from build123d import *

# Parameters (mm, degrees)
F0_W      = 1841.5
F0_H      = 622.3
F1_DEPTH  = 711.2
F2_W      = 1739.9
F2_H      = 609.6
F3_DEPTH  = 762
F4_W      = 520.7
F4_H      = 609.6
F5_DEPTH  = 2540
F6_W      = 1739.9
F6_H      = 520.7
F7_DEPTH  = 2540
F8_W      = 50.8
F8_H      = 50.8
F9_DEPTH  = 520.7
F10_W     = 50.8
F10_H     = 50.8
F11_DEPTH = 609.6
F12_W     = 50.8
F12_H     = 50.8
F13_DEPTH = 609.6


with BuildPart() as f1:
    # F0 (on Top) → F1 (new body)
    with BuildSketch(Plane.XY):
        with Locations((814.200432, 140.348346)):
            Rectangle(F0_W, F0_H)
    extrude(amount=F1_DEPTH)

    # F2 (on face) → F3 (cut)
    with BuildSketch(Plane.XZ.offset(170.801654)):
        with Locations((814.200432, 355.6)):
            Rectangle(F2_W, F2_H)
    extrude(amount=-F3_DEPTH, mode=Mode.SUBTRACT)

    # F4 (on face) → F5 (cut)
    with BuildSketch(Plane(origin=(-106.549568, 0, 0), x_dir=(0, -1, 0), z_dir=(-1, 0, 0))):
        with Locations((-140.348346, 355.6)):
            Rectangle(F4_W, F4_H)
    extrude(amount=-F5_DEPTH, mode=Mode.SUBTRACT)

    # F6 (on face) → F7 (cut)
    with BuildSketch(Plane.XY.offset(711.2)):
        with Locations((814.200432, 140.348346)):
            Rectangle(F6_W, F6_H)
    extrude(amount=-F7_DEPTH, mode=Mode.SUBTRACT)

    # F8 (on face) → F9 (join)
    with BuildSketch(Plane.XZ.offset(-400.698346)):
        with Locations((515.750432, 685.8)):
            Rectangle(F8_W, F8_H)
        with Locations((1112.650432, 685.8)):
            Rectangle(F8_W, F8_H)
    extrude(amount=F9_DEPTH)

    # F10 (on face) → F11 (join)
    with BuildSketch(Plane(origin=(0, 0, 660.4), x_dir=(1, 0, 0), z_dir=(0, 0, -1))):
        with Locations((1112.650432, -426.098346)):
            Rectangle(F10_W, F10_H)
        with Locations((515.750432, -426.098346)):
            Rectangle(F10_W, F10_H)
    extrude(amount=F11_DEPTH)

    # F12 (on face) → F13 (join)
    with BuildSketch(Plane(origin=(0, 0, 660.4), x_dir=(1, 0, 0), z_dir=(0, 0, -1))):
        with Locations((515.750432, 145.401654)):
            Rectangle(F12_W, F12_H)
        with Locations((1112.650432, 145.401654)):
            Rectangle(F12_W, F12_H)
    extrude(amount=F13_DEPTH)


solid = f1.part
Can you work these out from the model? Positions are in its coordinate system, mm. A direction names the side the tool comes from. Round coordinates to 2 decimals unless told otherwise and drop trailing zeros. Order: outer loops, then holes, each group sorted by start corner. A loop starts at its lowest first (then second) coordinate and runs counter-clockwise, first axis right, second up. Notation, with made-up numbers: M 85,15 L 103,15 A22 ccw 103,43 Z; hole C 23.5,35 d6. An arc over 180 degrees is marked long. Use a Markdown table: item, result.
1) If I drill on line 1 along Y through (x, z) = (1099, 393); line 2 along X through (y, z) = (280.5, 34); line 3 along Z through (x, y) = (1137, 257), over which ranges is the centre line in solid material (lowest first)?
Geometry says:
| item | result |
|---|---|
| line 1 | y = -170.8 to -120, 400.7 to 451.5 |
| line 2 | x = -106.55 to -55.75, 1684.15 to 1734.95 |
| line 3 | z = 660.4 to 711.2 |
2) Imagine slicing it at B-B (x = 1225). List the corners of the cut face in (y, z) for me, then the cut area to 3 significant figures.
Geometry says:
| item | result |
|---|---|
| outline | M -170.8,0 L -120,0 L -120,50.8 L -170.8,50.8 Z; M -170.8,660.4 L -120,660.4 L -120,711.2 L -170.8,711.2 Z; M 400.7,0 L 451.5,0 L 451.5,50.8 L 400.7,50.8 Z; M 400.7,660.4 L 451.5,660.4 L 451.5,711.2 L 400.7,711.2 Z |
| area | 10,300 mm² |
3) Imagine slicing it at C-C (z = 228.5). Give the number of separate pieces and of enclosed holes in the cut face, then the cut area to 3 significant figures.
Geometry says:
| item | result |
|---|---|
| separate pieces | 8 |
| enclosed holes | 0 |
| area | 20,600 mm² |
4) I'm going to push a flat-ended pin straight in: P1, Ø6, axis at x = 512.5, y = 248, coming from the -Z side. Where does the tip first touch, or does it pass through?
Geometry says:
| item | result |
|---|---|
| P1 | stops at z = 660.4 |
5) On a 3-axis mill with a long thin cutter (end or side, diameter ignored), from which of +Z, -Z, +X, -X, +Y, -Y can I reach the whole of each face in a straight line? I mean faces 1 (the face through (1709, 400.698, 351)), 2 (the face through (1138.05, 144, 685)), 3 (the face through (1684.15, -146, 351)). Say none if no direction works.
Geometry says:
| item | result |
|---|---|
| face 1 | +X, -X |
| face 2 | +Z, -Z |
| face 3 | +Y, -Y |
6) If we mould it in two halves opening along X, with no side actions, what happens to faces 4 (the face through (213, -145, 660.4)), 5 (the face through (-55.75, 137, 686)), 6 (the face through (-82, 400.698, 351))? For each: +X half, -X half, draft (parallel to the pull), parting line (faces both ways), or undercut.
Geometry says:
| item | result |
|---|---|
| face 4 | undercut |
| face 5 | undercut |
| face 6 | draft |
7) Imagine slicing it at A-A (y = 348). List the corners of the cut face in (x, z) for me, then the cut area to 3 significant figures.
Geometry says:
| item | result |
|---|---|
| outline | M -106.55,0 L -55.75,0 L -55.75,50.8 L -106.55,50.8 Z; M -106.55,660.4 L -55.75,660.4 L -55.75,711.2 L -106.55,711.2 Z; M 490.35,660.4 L 541.15,660.4 L 541.15,711.2 L 490.35,711.2 Z; M 1087.25,660.4 L 1138.05,660.4 L 1138.05,711.2 L 1087.25,711.2 Z; M 1684.15,0 L 1734.95,0 L 1734.95,50.8 L 1684.15,50.8 Z; M 1684.15,660.4 L 1734.95,660.4 L 1734.95,711.2 L 1684.15,711.2 Z |
| area | 15,500 mm² |
